```python
from build123d import *

# Parameters (mm, degrees)
CUT_EXTRUDE1_DEPTH   = 1.8
SHELL1_START         = -21.5
SHELL1_OUTLINE_R     = 3.65
SHELL1_DEPTH         = 21.5
SHELL1_START_2       = -13.25
SHELL1_2_OUTLINE_R   = 6.1
SHELL1_2_OUTLINE_R_2 = 3.65
SHELL1_2_DEPTH       = 4.85
SHELL1_START_3       = -8.4
SHELL1_3_OUTLINE_R   = 3.65
SHELL1_3_DEPTH       = 2.75
SHELL1_START_4       = -9.4
SHELL1_4_OUTLINE_R   = 6.6
SHELL1_4_OUTLINE_R_2 = 6.1
SHELL1_4_DEPTH       = 1
SHELL1_5_DEPTH       = 0.95
SHELL1_6_OUTLINE_R   = 6.6
SHELL1_6_OUTLINE_R_2 = 6.1
SHELL1_6_DEPTH       = 0.35
SKETCH3_R            = 3.766666667
CUT_EXTRUDE2_DEPTH   = 6.8


with BuildPart() as part:
    # Sketch1 → Revolve1 (revolve)
    with BuildSketch(Plane.XY, mode=Mode.PRIVATE) as revolve1_sk:
        Polygon((0, 0), (0, -22.5), (4.5, -22.5), (7.1, -14.25), (7.6, -14.25), (7.6, -11.9), (7.1, -11.9), (7.1, -10.4), (7.6, -10.4), (7.6, -7.4), (5.75, -7.4), (5.75, -4.65), (4.65, -4.65), (4.65, 0), align=None)
    revolve(revolve1_sk.sketch.rotate(Axis((0, 0, 0), (0, -1, 0)), 90), axis=Axis((0, 0, 0), (0, -1, 0)))

    # Sketch2 → Cut-Extrude1 (cut)
    with BuildSketch(Plane(origin=(0, -4.65, 0), x_dir=(1, 0, 0), z_dir=(0, 1, 0))):
        with BuildLine():
            Line((-4.75, -3.240370349), (-4.75, 3.240370349))
            ThreePointArc((-4.75, 3.240370349), (-5.75, 0), (-4.75, -3.240370349))
        make_face()
        with BuildLine():
            ThreePointArc((5.75, 0), (5.494315244, 1.695582496), (4.75, 3.240370349))
            Line((4.75, 3.240370349), (4.75, -3.240370349))
            ThreePointArc((4.75, -3.240370349), (5.494315244, -1.695582496), (5.75, 0))
        make_face()
    extrude(amount=-CUT_EXTRUDE1_DEPTH, mode=Mode.SUBTRACT)

    # Shell1: read off the stored shape, not the designer's step
    # Shell1 outline → Shell1 (cut)
    with BuildSketch(Plane(origin=(0, 0, 0), x_dir=(1, 0, 0), z_dir=(0, 1, 0)).offset(SHELL1_START)):
        Circle(SHELL1_OUTLINE_R)
    extrude(amount=SHELL1_DEPTH, mode=Mode.SUBTRACT)

    # Shell1 2 outline → Shell1 2 (cut)
    with BuildSketch(Plane(origin=(0, 0, 0), x_dir=(1, 0, 0), z_dir=(0, 1, 0)).offset(SHELL1_START_2)):
        Circle(SHELL1_2_OUTLINE_R)
        Circle(SHELL1_2_OUTLINE_R_2, mode=Mode.SUBTRACT)
    extrude(amount=SHELL1_2_DEPTH, mode=Mode.SUBTRACT)

    # Shell1 3 outline → Shell1 3 (cut)
    with BuildSketch(Plane(origin=(0, 0, 0), x_dir=(1, 0, 0), z_dir=(0, 1, 0)).offset(SHELL1_START_3)):
        with BuildLine():
            Line((3.75, -2.915475947), (3.75, 2.915475947))
            ThreePointArc((3.75, 2.915475947), (0, 4.75), (-3.75, 2.915475947))
            Line((-3.75, 2.915475947), (-3.75, -2.915475947))
            ThreePointArc((-3.75, -2.915475947), (0, -4.75), (3.75, -2.915475947))
        make_face()
        Circle(SHELL1_3_OUTLINE_R, mode=Mode.SUBTRACT)
    extrude(amount=SHELL1_3_DEPTH, mode=Mode.SUBTRACT)

    # Shell1 4 outline → Shell1 4 (cut)
    with BuildSketch(Plane(origin=(0, 0, 0), x_dir=(1, 0, 0), z_dir=(0, 1, 0)).offset(SHELL1_START_4)):
        Circle(SHELL1_4_OUTLINE_R)
        Circle(SHELL1_4_OUTLINE_R_2, mode=Mode.SUBTRACT)
    extrude(amount=SHELL1_4_DEPTH, mode=Mode.SUBTRACT)

    # Shell1 5 outline → Shell1 5 (cut)
    with BuildSketch(Plane(origin=(0, 0, 0), x_dir=(1, 0, 0), z_dir=(0, 1, 0)).offset(SHELL1_START_3)):
        with BuildLine():
            ThreePointArc((3.75, -2.915475947), (4.75, 0), (3.75, 2.915475947))
            Line((3.75, 2.915475947), (3.75, -2.915475947))
        make_face()
        with BuildLine():
            Line((-3.75, -2.915475947), (-3.75, 2.915475947))
            ThreePointArc((-3.75, 2.915475947), (-4.75, 0), (-3.75, -2.915475947))
        make_face()
    extrude(amount=SHELL1_5_DEPTH, mode=Mode.SUBTRACT)

    # Shell1 6 outline → Shell1 6 (cut)
    with BuildSketch(Plane(origin=(0, 0, 0), x_dir=(1, 0, 0), z_dir=(0, 1, 0)).offset(SHELL1_START_2)):
        Circle(SHELL1_6_OUTLINE_R)
        Circle(SHELL1_6_OUTLINE_R_2, mode=Mode.SUBTRACT)
    extrude(amount=SHELL1_6_DEPTH, mode=Mode.SUBTRACT)

    # Shell1 7 outline → Shell1 7 (revolve, cut)
    with BuildSketch(Plane.XY):
        Polygon((6.366666667, -13.25), (3.65, -13.25), (3.65, -21.5), (3.766666667, -21.5), align=None)
    revolve(axis=Axis((0, 0, 0), (0, 1, 0)), mode=Mode.SUBTRACT)

    # Sketch3 → Cut-Extrude2 (cut)
    with BuildSketch(Plane(origin=(0, -21.5, 0), x_dir=(1, 0, 0), z_dir=(0, 1, 0))):
        with Locations(Location((0, 0, 0), (0, 0, 270))):
            Circle(SKETCH3_R)
    extrude(amount=-CUT_EXTRUDE2_DEPTH, mode=Mode.SUBTRACT)


solid = part.part
```
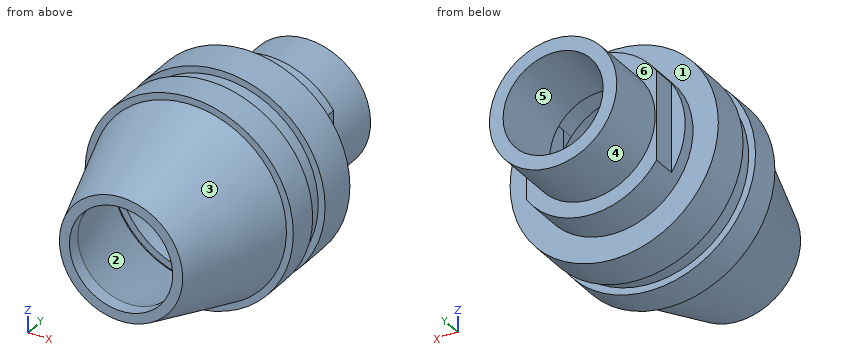
The model under review builds one solid part; all positions refer to its coordinate system, in mm. Face numbers are marked on the shaded views. A direction names the side the tool comes from. Coordinates: 2 decimals unless noted, no trailing zeros. Write each loop counter-clockwise with the first axis right and the second up, starting at its lowest first coordinate (ties: lowest second). Pieces come first, ordered by that corner, then holes. Notation, with made-up numbers: (17, 87) - (51, 87) arc R17 ccw to (51, 119) - close; hole circle Ø9 at (52, -3.75). An arc over 180 degrees is marked (long way). Write item = value, one per line.
(1) For line 1 (X direction, y = -11.1, z = 0); line 2 (Y direction, x = -4.5, z = 6); line 3 (Z direction, x = -0.25, y = -10.25), list the stretches that pass through material, from the lowest coordinate up. Write a range as [from, to].
Result sheet:
line_1 = [-7.1, -6.1], [6.1, 7.1]
line_2 = [-14.25, -11.9], [-10.4, -7.4]
line_3 = [-7.6, -6.09], [6.09, 7.6]
(2) Consider section B-B, the plane y = -7. Give the boundary of the cut face in (x, z), then the cut area to 3 significant figures.
Result sheet:
outline = circle Ø11.5 at (0, 0); hole (-3.75, -2.92) arc R4.75 ccw to (3.75, -2.92) - (3.75, 2.92) arc R4.75 ccw to (-3.75, 2.92) - close
area = 40.9 mm^2
(3) Consider section A-A, the plane y = -3.25. Give the boundary of the cut face in (x, z), then the cut area to 3 significant figures.
Result sheet:
outline = circle Ø9.3 at (0, 0); hole circle Ø7.3 at (0, 0)
area = 26.1 mm^2
(4) Mouldability with a two-part tool opening along Y and no side actions: class the marked faces 1, 2, 3 and 4 as pulls with the +Y half, pulls with the -Y half, needs draft (parallel to the pull), parting line crosses it, or undercut.
Result sheet:
face_1 = pulls with the +Y half
face_2 = undercut
face_3 = pulls with the -Y half
face_4 = needs draft
(5) For P1, Ø2, axis at x = -1.5, y = -16.5, coming from the +Z side; P2, Ø4, axis at x = 2, z = -3, coming from the -Y side; P3, Ø2, axis at y = -7.5, z = 3, coming from the -X side; P4, Ø2, axis at y = -5.5, z = 0, coming from the -X side, all flat-tipped, find the tip position at first contact; note any pin that passes through.
Result sheet:
P1 = 6.59
P2 = -22.5
P3 = -7.33
P4 = -5.75
(6) Consider section C-C, the plane y = -14. Give the boundary of the cut face in (x, z).
Result sheet:
outline = circle Ø15.2 at (0, 0); hole circle Ø12.26 at (0, 0)
(7) Machinability: for the marked faces 5 and 6, which of the approach directions +Z, -Z, +X, -X, +Y, -Y give a long, thin tool a straight path to every point of the face, cutting with its end or side? Answer none if there is none.
Result sheet:
face_5 = +Y, -Y
face_6 = +Y
